from build123d import *

# Parameters (mm, degrees)
SKETCH1_R           = 25
BOSS_EXTRUDE1_DEPTH = 5
SKETCH2_R           = 15
BOSS_EXTRUDE2_DEPTH = 95
BOSS_EXTRUDE4_DEPTH = 15
CUT_EXTRUDE1_DEPTH  = 20
SKETCH15_W          = 56
SKETCH15_H          = 21
CUT_EXTRUDE3_DEPTH  = 12
SKETCH17_R          = 2
SKETCH17_R_2        = 6.9
CUT_EXTRUDE4_DEPTH  = 5
SKETCH20_R          = 3
CUT_EXTRUDE5_DEPTH  = 2
SKETCH22_R          = 3
SKETCH22_R_2        = 1.5
CUT_EXTRUDE6_DEPTH  = 10
CUT_EXTRUDE7_DEPTH  = 3
SKETCH24_R          = 6.5
CUT_EXTRUDE8_DEPTH  = 3


with BuildPart() as part:
    # Sketch1 → Boss-Extrude1 (new body)
    with BuildSketch(Plane(origin=(0, 0, 0), x_dir=(1, 0, 0), z_dir=(0, 1, 0))):
        with Locations(Location((0, 0, 0), (0, 0, 270))):
            Circle(SKETCH1_R)
    extrude(amount=BOSS_EXTRUDE1_DEPTH)

    # Sketch2 → Boss-Extrude2 (add)
    with BuildSketch(Plane(origin=(0, 5, 0), x_dir=(1, 0, 0), z_dir=(0, 1, 0))):
        with Locations(Location((0, 0, 0), (0, 0, 270))):
            Circle(SKETCH2_R)
    extrude(amount=BOSS_EXTRUDE2_DEPTH)

    # Sketch5 → Boss-Extrude4 (add, symmetric)
    with BuildSketch(Plane(origin=(0, 100, 0), x_dir=(1, 0, 0), z_dir=(0, 1, 0))):
        with BuildLine():
            Line((75, 0), (15, 0))
            ThreePointArc((15, 0), (-10.606601718, -10.606601718), (0, 15))
            Line((0, 15), (75, 15))
            Line((75, 15), (75, 0))
        make_face()
    extrude(amount=BOSS_EXTRUDE4_DEPTH, both=True)

    # Sketch13 → Cut-Extrude1 (cut, symmetric)
    with BuildSketch(Plane(origin=(0, 0, 0), x_dir=(0, 0, -1), z_dir=(1, 0, 0))):
        with BuildLine():
            Line((4.957382287, 78.443263872), (4.957382287, 13.443263872))
            ThreePointArc((4.957382287, 13.443263872), (0, 8.485881586), (-4.957382287, 13.443263872))
            Line((-4.957382287, 13.443263872), (-4.957382287, 78.443263872))
            ThreePointArc((-4.957382287, 78.443263872), (0, 83.400646159), (4.957382287, 78.443263872))
        make_face()
    extrude(amount=CUT_EXTRUDE1_DEPTH, both=True, mode=Mode.SUBTRACT)

    # Sketch15 → Cut-Extrude3 (cut)
    with BuildSketch(Plane(origin=(0, 0, -15), x_dir=(-1, 0, 0), z_dir=(0, 0, -1))):
        with Locations((-44.68, 100.4)):
            Rectangle(SKETCH15_W, SKETCH15_H)
    extrude(amount=-CUT_EXTRUDE3_DEPTH, mode=Mode.SUBTRACT)

    # Sketch17 → Cut-Extrude4 (cut)
    with BuildSketch(Plane(origin=(0, 0, -3), x_dir=(-1, 0, 0), z_dir=(0, 0, -1))):
        with Locations((-68.98, 105.4)):
            Circle(SKETCH17_R)
        with Locations((-68.98, 95.4)):
            Circle(SKETCH17_R)
        with Locations((-20.18, 105.4)):
            Circle(SKETCH17_R)
        with Locations((-20.18, 95.4)):
            Circle(SKETCH17_R)
        with Locations((-55, 100)):
            Circle(SKETCH17_R_2)
    extrude(amount=-CUT_EXTRUDE4_DEPTH, mode=Mode.SUBTRACT)

    # Sketch20 → Cut-Extrude5 (cut)
    with BuildSketch(Plane.XY):
        with Locations((20.18, 105.4)):
            Circle(SKETCH20_R)
        with Locations((20.18, 95.4)):
            Circle(SKETCH20_R)
        with Locations((68.98, 105.4)):
            Circle(SKETCH20_R)
        with Locations((68.98, 95.4)):
            Circle(SKETCH20_R)
    extrude(amount=-CUT_EXTRUDE5_DEPTH, mode=Mode.SUBTRACT)

    # Sketch22 → Cut-Extrude6 (cut)
    with BuildSketch(Plane.XZ):
        with Locations(Location((0, 0, 0), (0, 0, 270))):
            Circle(SKETCH22_R)
        with Locations(Location((0, 16.5, 0), (0, 0, 270))):
            Circle(SKETCH22_R_2)
        with Locations(Location((0, -16.5, 0), (0, 0, 270))):
            Circle(SKETCH22_R_2)
    extrude(amount=-CUT_EXTRUDE6_DEPTH, mode=Mode.SUBTRACT)

    # Sketch23 → Cut-Extrude7 (cut)
    with BuildSketch(Plane.XZ):
        with BuildLine():
            Line((4.75, 15), (4.75, -15))
            ThreePointArc((4.75, -15), (0, -19.75), (-4.75, -15))
            Line((-4.75, -15), (-4.75, 15))
            ThreePointArc((-4.75, 15), (0, 19.75), (4.75, 15))
        make_face()
    extrude(amount=-CUT_EXTRUDE7_DEPTH, mode=Mode.SUBTRACT)

    # Sketch24 → Cut-Extrude8 (cut)
    with BuildSketch(Plane.XZ.offset(-3)):
        Circle(SKETCH24_R)
    extrude(amount=CUT_EXTRUDE8_DEPTH, mode=Mode.SUBTRACT)


solid = part.part
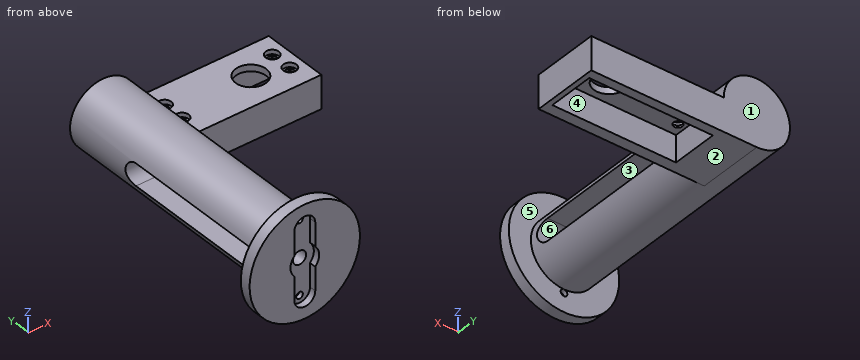
Here's how the part is built. I have some questions about the finished solid (model axes, mm). Face numbers are marked on the shaded views. A direction names the side the tool comes from. Round coordinates to 2 decimals unless told otherwise and drop trailing zeros. Order: outer loops, then holes, each group sorted by start corner. A loop starts at its lowest first (then second) coordinate and runs counter-clockwise, first axis right, second up. Notation, with made-up numbers: M 20.5,-40 L 61.5,-40 A20 ccw 61.5,-2 Z; hole C 54,-39.75 d3. An arc over 180 degrees is marked long. Return JSON: item names as keys, results as strings. Group by question number.
1. If we section it at C-C on z = -11.5: List the corners of the cut face in (x, y) for me, then the cut area to 3 significant figures.
2. If we mould it in two halves opening along Z, with no side actions, what happens to the marked faces 1, 2 and 3? For each: pulls with the +Z half, pulls with the -Z half, needs draft (parallel to the pull), parting line crosses it, or undercut.
3. I'm going to push flat-ended pins straight in: pin 1 Ø5 at (x, y) = (20.18, 95.4) entering from +Z; pin 2 Ø12 at (x, z) = (30.5, -8) entering from -Y; pin 3 Ø8 at (x, y) = (11.5, 20.5) entering from -Z; pin 4 Ø3.5 at (x, y) = (20.18, 105.4) entering from -Z. Where does each tip first touch, or does it pass through?
4. If we section it at B-B on y = 100: List the corners of the cut face in (x, z) for me, then the cut area to 3 significant figures.
5. If we section it at D-D on x = 45: List the corners of the cut face in (y, z) for me.
6. If we section it at A-A on x = 55: List the corners of the cut face in (y, z) for me, then the cut area to 3 significant figures.
7. On a 3-axis mill with a long thin cutter (end or side, diameter ignored), from which of +Z, -Z, +X, -X, +Y, -Y can I reach the whole of each face in a straight line? I mean the marked faces 4, 5 and 6. Say none if no direction works.
8. Please list where these lines run through material, in increasing order: probe 1 along Y at (x, z) = (20.18, -2.6); probe 2 along Y at (x, z) = (20, -1); probe 3 along Y at (x, z) = (68.98, -1).
Reply:
{
 "1": {"outline": "M -22.2,0 L -4.75,0 L -4.75,3 L 4.75,3 L 4.75,0 L 22.2,0 L 22.2,5 L 9.63,5 L 9.63,85 L 75,85 L 75,115 L -9.63,115 L -9.63,5 L -22.2,5 Z; hole M 16.68,89.9 L 72.68,89.9 L 72.68,110.9 L 16.68,110.9 Z", "area": "3,100 mm^2"},
 "2": {"face 1": "needs draft", "face 2": "pulls with the -Z half", "face 3": "undercut"},
 "3": {"pin 1": "z = -2", "pin 2": "y = 85", "pin 3": "z = -12.99", "pin 4": "through"},
 "4": {"outline": "M 0,-15 L 16.68,-15 L 16.68,-3 L 48.1,-3 L 48.1,0 L 15,0 A15 ccw long Z; M 61.9,-3 L 72.68,-3 L 72.68,-15 L 75,-15 L 75,0 L 61.9,0 Z", "area": "942 mm^2"},
 "5": {"outline": "M 85,-15 L 89.9,-15 L 89.9,-3 L 110.9,-3 L 110.9,-15 L 115,-15 L 115,0 L 85,0 Z"},
 "6": {"outline": "M 85,-15 L 89.9,-15 L 89.9,-3 L 93.1,-3 L 93.1,0 L 85,0 Z; M 106.9,-3 L 110.9,-3 L 110.9,-15 L 115,-15 L 115,0 L 106.9,0 Z", "area": "157 mm^2"},
 "7": {"face 4": "-Z", "face 5": "none", "face 6": "+X, -X"},
 "8": {"probe 1": "0 to 5, 85 to 93.4, 97.4 to 103.4, 107.4 to 115", "probe 2": "0 to 5, 85 to 92.41, 98.39 to 102.41, 108.39 to 115", "probe 3": "85 to 92.4, 98.4 to 102.4, 108.4 to 115"}
}
